```python
from build123d import *

# Parameters (mm, degrees)
BOSS_EXTRUDE1_DEPTH      = 8
BOSS_EXTRUDE1_DEPTH_BACK = 8
SKETCH2_R                = 95
CUT_EXTRUDE1_DEPTH       = 4
CUT_EXTRUDE1_DEPTH_BACK  = 4
SKETCH2_5_R              = 95
SKETCH2_5_R_2            = 89
SKETCH7_R                = 4.5
CUT_EXTRUDE2_DEPTH       = 167
SKETCH3_R                = 33.75
CUT_EXTRUDE3_DEPTH       = 43
CUT_EXTRUDE4_DEPTH       = 112
CUT_EXTRUDE4_DEPTH_BACK  = 60
SKETCH10_R               = 4.5


with BuildPart() as part:
    # Sketch2 → Boss-Extrude1 (new, two sides: drawn at the far end of the back side and taken through both)
    with BuildSketch(Plane.XY.offset(-BOSS_EXTRUDE1_DEPTH_BACK)):
        Circle(SKETCH2_R)
    extrude(amount=BOSS_EXTRUDE1_DEPTH + BOSS_EXTRUDE1_DEPTH_BACK)

    # Sketch2_5 → Cut-Extrude1 (cut, two sides: drawn at the far end of the back side and taken through both)
    with BuildSketch(Plane.XY.offset(-CUT_EXTRUDE1_DEPTH_BACK)):
        Circle(SKETCH2_5_R)
        Circle(SKETCH2_5_R_2, mode=Mode.SUBTRACT)
    extrude(amount=CUT_EXTRUDE1_DEPTH + CUT_EXTRUDE1_DEPTH_BACK, mode=Mode.SUBTRACT)

    # Sketch7 → Cut-Extrude2 (cut)
    with BuildSketch(Plane.XY.offset(8)):
        with Locations((-50, -48.75)):
            Circle(SKETCH7_R)
        with Locations((50, -48.75)):
            Circle(SKETCH7_R)
        with Locations((-25, -48.75)):
            Circle(SKETCH7_R)
    extrude(amount=-CUT_EXTRUDE2_DEPTH, mode=Mode.SUBTRACT)

    # Sketch3 → Cut-Extrude3 (cut)
    with BuildSketch(Plane.XY.offset(8)):
        Circle(SKETCH3_R)
    extrude(amount=-CUT_EXTRUDE3_DEPTH, mode=Mode.SUBTRACT)

    # Sketch10 → Cut-Extrude4 (cut, two sides: drawn at the far end of the back side and taken through both)
    with BuildSketch(Plane(origin=(0, 0, -8), x_dir=(-1, 0, 0), z_dir=(0, 0, -1)).offset(-CUT_EXTRUDE4_DEPTH_BACK)):
        with Locations(Location((0, 70, 0), (0, 0, 180))):
            Circle(SKETCH10_R)
    extrude(amount=CUT_EXTRUDE4_DEPTH + CUT_EXTRUDE4_DEPTH_BACK, mode=Mode.SUBTRACT)


solid = part.part
```
Geometry check sheet. Reference: the model listing, model coordinates, mm. A direction names the side the tool comes from. Give positions to 0.01 mm unless a question says otherwise; leave off trailing zeros. Loops run counter-clockwise (first coordinate to the right, second up) from the corner with the lowest first, then second, coordinate; pieces in that order, holes last. Notation, with made-up numbers: (-17.75, 9) - (-13.75, 9) arc R12 cw to (-13.75, 32) - close; hole circle Ø7 at (73.5, 56.25). An arc over 180 degrees is marked (long way). Use CSV: the item, a comma, the result in double quotes. Start each with the question number.
Q1. Section check D-D, the plane x = -50. Record the cut outline in (y, z).
Q2. Section check C-C, the plane y = -48.75. Record the cut outline in (x, z).
Q3. Scan lines: probe 1 along Y at (x, z) = (0, 4.5); probe 2 along Z at (x, y) = (39, -83); probe 3 along X at (y, z) = (-0.5, 3). Record each from-to range of solid material in increasing order. Write a range as from..to.
Q4. Release check for a two-part mould opening along Z. For faces 3 (the face through (-85, -28, 4)), 4 (the face through (-26.78, -20.54, 0.11)), 5 (the face through (41, 1, 8)), 6 (the face through (-65.597, 60.15, -0.056)) record: +Z half, -Z half, draft (parallel to the pull), parting line (faces both ways), or undercut.
Q5. Access from +Z, -Z, +X, -X, +Y, -Y to the whole of each face (thin tool, end or side, straight path). Record for faces 1 (the face through (-85, -28, -4)), 2 (the face through (52.08, -52.74, 0.11)).
Q6. Section check A-A, the plane y = 0. Record the cut outline in (x, z).
Q7. Section check B-B, the plane x = 0. Record the cut outline in (y, z), and give its area (3 significant figures).
Q8. Go/stop test with flat-tipped pins: pin 1 Ø2 at (x, z) = (-11, 4.5) entering from +Y; pin 2 Ø8 at (y, z) = (14.5, 5) entering from -X; pin 3 Ø3 at (x, z) = (-61.5, 0) entering from -Y; pin 4 Ø7 at (x, y) = (-25, -48.75) entering from +Z. Record where each tip stops, or that it passes through.
Findings below:
1,outline,"(-80.78, -8) - (-53.25, -8) - (-53.25, 8) - (-80.78, 8) - (-80.78, 4) - (-73.63, 4) - (-73.63, -4) - (-80.78, -4) - close; (-44.25, -8) - (80.78, -8) - (80.78, -4) - (73.63, -4) - (73.63, 4) - (80.78, 4) - (80.78, 8) - (-44.25, 8) - close"
2,outline,"(-81.54, -8) - (-54.5, -8) - (-54.5, 8) - (-81.54, 8) - (-81.54, 4) - (-74.46, 4) - (-74.46, -4) - (-81.54, -4) - close; (-45.5, -8) - (-29.5, -8) - (-29.5, 8) - (-45.5, 8) - close; (-20.5, -8) - (45.5, -8) - (45.5, 8) - (-20.5, 8) - close; (54.5, -8) - (81.54, -8) - (81.54, -4) - (74.46, -4) - (74.46, 4) - (81.54, 4) - (81.54, 8) - (54.5, 8) - close"
3,probe 1,"y = -95..-33.75, 33.75..65.5, 74.5..95"
3,probe 2,"z = -8..-4, 4..8"
3,probe 3,"x = -89..-33.75, 33.75..89"
4,face 3,"undercut"
4,face 4,"draft"
4,face 5,"+Z half"
4,face 6,"undercut"
5,face 1,"none"
5,face 2,"+Z, -Z"
6,outline,"(-95, -8) - (-33.75, -8) - (-33.75, 8) - (-95, 8) - (-95, 4) - (-89, 4) - (-89, -4) - (-95, -4) - close; (33.75, -8) - (95, -8) - (95, -4) - (89, -4) - (89, 4) - (95, 4) - (95, 8) - (33.75, 8) - close"
7,outline,"(-95, -8) - (-33.75, -8) - (-33.75, 8) - (-95, 8) - (-95, 4) - (-89, 4) - (-89, -4) - (-95, -4) - close; (33.75, -8) - (65.5, -8) - (65.5, 8) - (33.75, 8) - close; (74.5, -8) - (95, -8) - (95, -4) - (89, -4) - (89, 4) - (95, 4) - (95, 8) - (74.5, 8) - close"
7,area,"1,720 mm^2"
8,pin 1,"stops at y = 94.47"
8,pin 2,"stops at x = -94.42"
8,pin 3,"stops at y = -65.73"
8,pin 4,"passes through"
